Model file for the job. Use its own axes, mm. Coordinates: 2 decimals unless noted, no trailing zeros. Loops run counter-clockwise (first coordinate to the right, second up) from the corner with the lowest first, then second, coordinate; pieces in that order, holes last.
Autodesk Inventor part; units mm, degrees
ref_plane "YZ Plane" through (0, 0, 0) normal (1, 0, 0) x (0, 1, 0)
ref_plane "XZ Plane" through (0, 0, 0) normal (0, 1, 0) x (-1, 0, 0)
ref_plane "XY Plane" through (0, 0, 0) normal (0, 0, 1) x (1, 0, 0)
sketch "Sketch1" plane through (0, 0, 0) normal (0, 0, 1) x (1, 0, 0)
  circle A0 centre (0, 0) radius 6.604
  arc A1 (-6.5253, -6.9387) -> (-4.4452, 8.4241) centre (0, 0) ccw
  line L0 (0, 27.271) -> (-20.415, -4.6403)
  line L1 (-20.415, -4.6403) -> (0, -73.9689)
  arc A2 (0, 27.271) -> (-4.4452, 8.4241) centre (172.4432, -23.349) ccw
  arc A3 (-6.5253, -6.9387) -> (0, -73.9689) centre (172.4432, -23.349) ccw
  dimension "d0" = 13.208
  dimension "d1" = 19.05
extrude "Extrusion1" add sketch "Sketch1" along normal blind 5.08
sketch "Sketch2" plane through (0, 0, 0) normal (1, 0, 0) x (0, 1, 0)
  line L0 (-73.9689, 0) -> (-73.9689, 5.08)
  line L1 (-73.9689, 2.54) -> (-0.7706, 7.6585)
  line L2 (-0.7706, 7.6585) -> (-0.7706, -2.5785)
  line L3 (-0.7706, -2.5785) -> (-73.9689, 2.54)
  line L4 (-0.7706, -2.5785) -> (-76.3846, -2.5785)
  line L5 (-76.3846, -2.5785) -> (-76.3846, 10.5273)
  line L6 (-76.3846, 10.5273) -> (-0.7706, 10.5273)
  line L7 (-0.7706, 10.5273) -> (-0.7706, 7.6585)
  point P0 (0, 0)
  dimension "d4" = 86
  dimension "d5" = 86
extrude "Extrusion2" cut sketch "Sketch2" against normal blind 25.7175 contours L3 L4 L5 L6 L7 L1
sketch "Sketch3" plane through (0, 0, 0) normal (1, 0, 0) x (0, 1, 0)
  line L0 (8.4241, 0) -> (27.271, 0)
  line L1 (15.3537, 0) -> (15.3537, 5.0379)
  circle A0 centre (15.3537, 2.519) radius 1.27
  point P0 (0, 0)
  dimension "d8" = 2.54
extrude "Extrusion3" cut sketch "Sketch3" against normal blind 25.7175
sketch "Sketch4" plane through (0, 0, 0) normal (0, 1, 0) x (-1, 0, 0)
  line L0 (20.415, 0) -> (20.415, 5.08)
  line L1 (6.5253, 5.08) -> (-9.525, 5.08)
  point P0 (0, 0)
  point P1 (4.4452, 5.08)
  dimension "d11" = 29.94
properties part number "legV2"
Q1. Flat gauge pins, fed straight in: P1, Ø1, axis at y = -30, z = 3, coming from the +X side; P2, Ø2, axis at y = -36.5, z = 1, coming from the -X side; P3, Ø3, axis at y = 15.35, z = 2.52, coming from the +X side. Where does each tip first touch, or does it go through?
Answers:
P1: stops at x = -7.13
P2: stops at x = -11.33
P3: stops at x = -2.72
Q2. Slice it at C-C (x = -14). List the corners of the cut face in (y, z).
Answers:
outline: (-26.43, 0) - (5.39, 0) - (5.39, 5.08) - (-26.43, 5.08) - close
Q3. Slice it at B-B (x = 1.75). List the corners of the cut face in (y, z), and give its area (3 significant figures).
Answers:
outline: (-9.36, 0) - (-6.37, 0) - (-6.37, 5.08) - (-9.36, 5.08) - close; (6.37, 0) - (9.36, 0) - (9.36, 5.08) - (6.37, 5.08) - close
area: 30.4 mm2
Q4. Mould opens along Y. For faces 1 (the flat face through (-10.065, 11.539, 2.504)), 2 (the cylindrical face through (9.474, -0.988, 2.504)), 3 (the flat face through (-6.91, -47.65, 0.7)), 4 (the flat face through (-8, -7, 0)) say: +Y half, -Y half, draft (parallel to the pull), parting line (faces both ways), or undercut.
Answers:
face 1: +Y half
face 2: undercut
face 3: -Y half
face 4: draft
Q5. Drill centre lines: line 1 (Y direction, x = -5, z = 0.9); line 2 (X direction, y = 2, z = 2); line 3 (Y direction, x = 6, z = 3.55). Where is each one in solid material? Low to high.
Answers:
line 1: y = -8.11 to -4.31, 4.31 to 19.46
line 2: x = -16.17 to -6.29, 6.29 to 9.31
line 3: y = -7.4 to -2.76, 2.76 to 7.4
Q6. Slice it at A-A (y = 0). List the corners of the cut face in (x, z), and give its area (3 significant figures).
Answers:
outline: (-17.45, 0) - (-6.6, 0) - (-6.6, 5.08) - (-17.45, 5.08) - close; (6.6, 0) - (9.52, 0) - (9.52, 5.08) - (6.6, 5.08) - close
area: 69.9 mm2
